Geometry: final body of the model. Coordinates: model frame, mm. Coordinates: 2 decimals unless noted, no trailing zeros. Order: outer loops, then holes, each group sorted by start corner. A loop starts at its lowest first (then second) coordinate and runs counter-clockwise, first axis right, second up. Notation, with made-up numbers: (46.5, 3.25) -> (102.5, 3.25) arc R22 cw to (102.5, 11.25) -> close; hole circle Ø6 at (20.25, -8). An arc over 180 degrees is marked (long way). Use one line per item in the form item = value.
Autodesk Fusion 360 part; units mm, degrees
sketch "Dog_body" plane through (0, 0, 0) normal (0, 0, 1) x (1, 0, 0)
  line L0 (-5.9546, 3.7769) -> (-5.6, 3.7769)
  line L1 (-5.6, 3.7769) -> (-5.6, 4.1551)
  line L2 (-5.6, 4.1551) -> (-5.2, 4.1551)
  line L3 (-5.2, 4.1551) -> (-5.2, 4.6)
  line L4 (-5.2, 4.6) -> (-4.8, 4.6)
  line L5 (-4.8, 4.6) -> (-4.8, 5)
  line L6 (-4.8, 5) -> (-4.0585, 5)
  line L7 (-4.0585, 5) -> (-4.0585, 5.4)
  line L8 (-4.0585, 5.4) -> (-2.4, 5.4)
  line L9 (-2.4, 5.4) -> (-2.4, 5)
  line L10 (-2.4, 5) -> (-0.4, 5)
  line L11 (-0.4, 5) -> (-0.4, 4.6)
  line L12 (-5.9546, 3.7769) -> (-5.9546, 2.2)
  line L13 (-5.9546, 2.2) -> (-5.6, 2.2)
  line L14 (-5.6, 2.2) -> (-5.6, 1.4)
  line L15 (-5.6, 1.4) -> (-5.9546, 1.4)
  line L16 (-5.9546, 1.4) -> (-5.9546, 0.2)
  line L17 (-5.9546, 0.2) -> (-5.6, 0.2)
  line L18 (-5.6, 0.2) -> (-5.6, -0.2)
  line L19 (-5.6, -0.2) -> (-4.8, -0.2)
  line L20 (-4.8, -0.2) -> (-4.8, -0.7)
  line L21 (-4.8, -0.7) -> (-3.6, -0.7)
  line L22 (-3.6, -0.7) -> (-3.6, -1.9)
  line L23 (-3.6, -1.9) -> (-3.2, -1.9)
  line L24 (-3.2, -1.9) -> (-3.2, -3)
  line L25 (-3.2, -3) -> (-3.6, -3)
  line L26 (-3.6, -3) -> (-3.6, -3.7529)
  line L27 (-3.6, -3.7529) -> (-4.1, -3.7529)
  line L28 (-4.1, -3.7529) -> (-4.1, -4.6)
  line L29 (-4.1, -4.6) -> (-2.4, -4.6)
  line L30 (-2.4, -4.6) -> (-2.4, -4.1765)
  line L31 (-2.4, -4.1765) -> (-1.9, -4.1765)
  line L32 (-1.9, -4.1765) -> (-1.9, -3.4)
  line L33 (-1.9, -3.4) -> (-1.1, -3.4)
  line L34 (-1.1, -3.4) -> (-1.1, -4.1765)
  line L35 (-1.1, -4.1765) -> (-1.6, -4.1765)
  line L36 (-1.6, -4.1765) -> (-1.6, -5)
  line L37 (-1.6, -5) -> (-0.1, -5)
  line L38 (-0.1, -5) -> (-0.1, -4.5882)
  line L39 (-0.1, -4.5882) -> (0.5, -4.5882)
  line L40 (0.5, -4.5882) -> (0.5, -3.8)
  line L41 (5.1495, 3.3539) -> (5.1495, 1.4)
  line L42 (5.1495, 1.4) -> (4.8, 1.4)
  line L43 (4.8, 1.4) -> (4.8, 1)
  line L44 (4.8, 1) -> (5.1495, 1)
  line L45 (5.1495, 1) -> (5.1495, 0.2)
  line L46 (5.1495, 0.2) -> (5.5479, 0.2)
  line L47 (5.5479, 0.2) -> (5.5479, -1)
  line L48 (5.5479, -1) -> (5.9, -1)
  line L49 (5.9, -1) -> (5.9, -3.4)
  line L50 (-0.4, 4.6) -> (0, 4.6)
  line L51 (0, 4.6) -> (0, 4.2)
  line L52 (0, 4.2) -> (0.4, 4.2)
  line L53 (0.4, 4.2) -> (0.4, 3.8)
  line L54 (0.4, 3.8) -> (0.8, 3.8)
  line L55 (0.8, 3.8) -> (0.8, 3.4)
  line L56 (0.8, 3.4) -> (1.2, 3.4)
  line L57 (1.2, 3.4) -> (1.2, 1.8)
  line L58 (1.2, 1.8) -> (0.8, 1.8)
  line L59 (0.8, 1.8) -> (0.8, 1.4)
  line L60 (0.8, 1.4) -> (0.4, 1.4)
  line L61 (0.4, 1.4) -> (0.4, 1)
  line L62 (0.4, 1) -> (1.1786, 1)
  line L63 (1.1786, 1) -> (1.1786, 1.4)
  line L64 (1.1786, 1.4) -> (1.9689, 1.4)
  line L65 (1.9689, 1.4) -> (1.9689, 1.8)
  line L66 (1.9689, 1.8) -> (3.6, 1.8)
  line L67 (3.6, 1.8) -> (3.6, 2.2)
  line L68 (3.6, 2.2) -> (4, 2.2)
  line L69 (4, 2.2) -> (4, 3.3596)
  line L70 (4, 3.3596) -> (3.5503, 3.3596)
  line L71 (3.5503, 3.3596) -> (3.5503, 4.2)
  line L72 (3.5503, 4.2) -> (3.2, 4.2)
  line L73 (3.2, 4.2) -> (3.2, 5)
  line L74 (3.2, 5) -> (4, 5)
  line L75 (4, 5) -> (4, 4.6)
  line L76 (4, 4.6) -> (4.4, 4.6)
  line L77 (4.4, 4.6) -> (4.4, 4.2)
  line L78 (4.4, 4.2) -> (4.7373, 4.2)
  line L79 (4.7373, 4.2) -> (4.7373, 3.4)
  line L80 (4.7373, 3.4) -> (4.7373, 3.3539)
  line L81 (4.7373, 3.3539) -> (5.1495, 3.3539)
  line L82 (0.5, -3.8) -> (0.8, -3.8)
  line L83 (0.8, -3.8) -> (0.8, -3)
  line L84 (0.8, -3) -> (1.5654, -3)
  line L85 (1.5654, -3) -> (1.5654, -3.5)
  line L86 (1.5654, -3.5) -> (3.2, -3.5)
  line L87 (3.2, -3.5) -> (3.2, -2.6)
  line L88 (3.2, -2.6) -> (3.6, -2.6)
  line L89 (3.6, -2.6) -> (3.6, -2.2)
  line L90 (3.6, -2.2) -> (4.3564, -2.2)
  line L91 (4.3564, -2.2) -> (4.3564, -2.9)
  line L92 (4.3564, -2.9) -> (3.9, -2.9)
  line L93 (3.9, -2.9) -> (3.9, -3.8)
  line L94 (3.9, -3.8) -> (5.5, -3.8)
  line L95 (5.5, -3.4) -> (5.9, -3.4)
  line L96 (5.5, -3.4) -> (5.5, -3.8)
extrude "Extrude1" add sketch "Dog_body" along normal blind 0.5
sketch "Dog_eyes" plane through (0, 0, 0.5) normal (0, 0, 1) x (-1, 0, 0)
  line L0 (5.9546, -3.7769) -> (5.9546, -2.2)
  line L1 (5.9546, -2.2) -> (5.6, -2.2)
  line L2 (5.6, -2.2) -> (5.6, -1.4)
  line L3 (5.6, -1.4) -> (5.9546, -1.4)
  line L4 (5.9546, -1.4) -> (5.9546, -0.2)
  line L5 (5.9546, -0.2) -> (5.6, -0.2)
  line L6 (5.6, -0.2) -> (5.6, 0.2)
  line L7 (5.6, 0.2) -> (4.8, 0.2)
  line L8 (4.8, 0.2) -> (4.8, 0.7)
  line L9 (4.8, 0.7) -> (3.6, 0.7)
  line L10 (3.6, 0.7) -> (3.6, 1.9)
  line L11 (3.6, 1.9) -> (3.2, 1.9)
  line L12 (3.2, 1.9) -> (3.2, 3)
  line L13 (3.2, 3) -> (3.6, 3)
  line L14 (3.6, 3) -> (3.6, 3.7529)
  line L15 (3.6, 3.7529) -> (4.1, 3.7529)
  line L16 (4.1, 3.7529) -> (4.1, 4.6)
  line L17 (4.1, 4.6) -> (2.4, 4.6)
  line L18 (2.4, 4.6) -> (2.4, 4.1765)
  line L19 (2.4, 4.1765) -> (1.9, 4.1765)
  line L20 (1.9, 4.1765) -> (1.9, 3.4)
  line L21 (1.9, 3.4) -> (1.1, 3.4)
  line L22 (1.1, 3.4) -> (1.1, 4.1765)
  line L23 (1.1, 4.1765) -> (1.6, 4.1765)
  line L24 (1.6, 4.1765) -> (1.6, 5)
  line L25 (1.6, 5) -> (0.1, 5)
  line L26 (0.1, 5) -> (0.1, 4.5882)
  line L27 (0.1, 4.5882) -> (-0.5, 4.5882)
  line L28 (-0.5, 4.5882) -> (-0.5, 3.8)
  line L29 (-0.5, 3.8) -> (-0.8, 3.8)
  line L30 (-0.8, 3.8) -> (-0.8, 3)
  line L31 (-0.8, 3) -> (-1.5654, 3)
  line L32 (-1.5654, 3) -> (-1.5654, 3.5)
  line L33 (-1.5654, 3.5) -> (-3.2, 3.5)
  line L34 (-3.2, 3.5) -> (-3.2, 2.6)
  line L35 (-3.2, 2.6) -> (-3.6, 2.6)
  line L36 (-3.6, 2.6) -> (-3.6, 2.2)
  line L37 (-3.6, 2.2) -> (-4.3564, 2.2)
  line L38 (-4.3564, 2.2) -> (-4.3564, 2.9)
  line L39 (-4.3564, 2.9) -> (-3.9, 2.9)
  line L40 (-3.9, 2.9) -> (-3.9, 3.8)
  line L41 (-3.9, 3.8) -> (-5.5, 3.8)
  line L42 (-5.5, 3.8) -> (-5.5, 3.4)
  line L43 (-5.5, 3.4) -> (-5.9, 3.4)
  line L44 (-5.9, 3.4) -> (-5.9, 1)
  line L45 (-5.9, 1) -> (-5.5479, 1)
  line L46 (-5.5479, 1) -> (-5.5479, -0.2)
  line L47 (-5.5479, -0.2) -> (-5.1495, -0.2)
  line L48 (-5.1495, -0.2) -> (-5.1495, -1)
  line L49 (-5.1495, -1) -> (-4.8, -1)
  line L50 (-4.8, -1) -> (-4.8, -1.4)
  line L51 (-4.8, -1.4) -> (-5.1495, -1.4)
  line L52 (-5.1495, -1.4) -> (-5.1495, -3.3539)
  line L53 (-5.1495, -3.3539) -> (-4.7373, -3.3539)
  line L54 (-4.7373, -3.3539) -> (-4.7373, -4.2)
  line L55 (-4.7373, -4.2) -> (-4.4, -4.2)
  line L56 (-4.4, -4.2) -> (-4.4, -4.6)
  line L57 (-4.4, -4.6) -> (-4, -4.6)
  line L58 (-4, -4.6) -> (-4, -5)
  line L59 (-4, -5) -> (-3.2, -5)
  line L60 (-3.2, -5) -> (-3.2, -4.2)
  line L61 (-3.2, -4.2) -> (-3.5503, -4.2)
  line L62 (-3.5503, -4.2) -> (-3.5503, -3.3596)
  line L63 (-3.5503, -3.3596) -> (-4, -3.3596)
  line L64 (-4, -3.3596) -> (-4, -2.2)
  line L65 (-4, -2.2) -> (-3.6, -2.2)
  line L66 (-3.6, -2.2) -> (-3.6, -1.8)
  line L67 (-3.6, -1.8) -> (-1.9689, -1.8)
  line L68 (-1.9689, -1.8) -> (-1.9689, -1.4)
  line L69 (-1.9689, -1.4) -> (-1.1786, -1.4)
  line L70 (-1.1786, -1.4) -> (-1.1786, -1)
  line L71 (-1.1786, -1) -> (-0.4, -1)
  line L72 (-0.4, -1) -> (-0.4, -1.4)
  line L73 (-0.4, -1.4) -> (-0.8, -1.4)
  line L74 (-0.8, -1.4) -> (-0.8, -1.8)
  line L75 (-0.8, -1.8) -> (-1.2, -1.8)
  line L76 (-1.2, -1.8) -> (-1.2, -3.4)
  line L77 (-1.2, -3.4) -> (-0.8, -3.4)
  line L78 (-0.8, -3.4) -> (-0.8, -3.8)
  line L79 (-0.8, -3.8) -> (-0.4, -3.8)
  line L80 (-0.4, -3.8) -> (-0.4, -4.2)
  line L81 (-0.4, -4.2) -> (0, -4.2)
  line L82 (0, -4.2) -> (0, -4.6)
  line L83 (0, -4.6) -> (0.4, -4.6)
  line L84 (0.4, -4.6) -> (0.4, -5)
  line L85 (0.4, -5) -> (2.4, -5)
  line L86 (2.4, -5) -> (2.4, -5.4)
  line L87 (2.4, -5.4) -> (4.0585, -5.4)
  line L88 (4.0585, -5.4) -> (4.0585, -5)
  line L89 (4.0585, -5) -> (4.8, -5)
  line L90 (4.8, -5) -> (4.8, -4.6)
  line L91 (4.8, -4.6) -> (5.2, -4.6)
  line L92 (5.2, -4.6) -> (5.2, -4.1551)
  line L93 (5.2, -4.1551) -> (5.6, -4.1551)
  line L94 (5.6, -4.1551) -> (5.6, -3.7769)
  line L95 (5.6, -3.7769) -> (5.9546, -3.7769)
  line L96 (3.2, -3) -> (3.2, -2)
  line L97 (3.2, -2) -> (2.6, -2)
  line L98 (2.6, -2) -> (2.6, -3)
  line L99 (2.6, -3) -> (3.2, -3)
  line L100 (5.2, -3.3) -> (5.2, -2.5)
  line L101 (5.2, -2.5) -> (4.8, -2.5)
  line L102 (4.8, -2.5) -> (4.8, -3.4)
  line L103 (4.8, -3.4) -> (5.2, -3.4)
  line L104 (5.2, -3.4) -> (5.2, -3.3)
extrude "Extrude2" cut sketch "Dog_eyes" against normal blind 0.2 contours L96 L97 L98 L99 | L100 L101 L102 L103 L104
sketch "Sketch3" plane through (0, 0, 0.5) normal (0, 0, 1) x (-1, 0, 0)
  line L0 (4.8, -2.5) -> (5.2, -2.5)
  line L1 (5.2, -2.5) -> (5.2, -3.4)
  line L2 (5.2, -3.4) -> (4.8, -3.4)
  line L3 (4.8, -3.4) -> (4.8, -2.5)
  line L4 (3.2, -2) -> (3.2, -3)
  line L5 (3.2, -3) -> (2.6, -3)
  line L6 (2.6, -3) -> (2.6, -2)
  line L7 (2.6, -2) -> (3.2, -2)
  line L8 (5.9546, -3.7769) -> (5.9546, -2.2)
  line L9 (5.9546, -2.2) -> (5.6, -2.2)
  line L10 (5.6, -2.2) -> (5.6, -1.4)
  line L11 (5.6, -1.4) -> (5.9546, -1.4)
  line L12 (5.9546, -1.4) -> (5.9546, -0.2)
  line L13 (5.9546, -0.2) -> (5.6, -0.2)
  line L14 (5.6, -0.2) -> (5.6, 0.2)
  line L15 (5.6, 0.2) -> (4.8, 0.2)
  line L16 (4.8, 0.2) -> (4.8, 0.7)
  line L17 (4.8, 0.7) -> (3.6, 0.7)
  line L18 (3.6, 0.7) -> (3.6, 1.9)
  line L19 (3.6, 1.9) -> (3.2, 1.9)
  line L20 (3.2, 1.9) -> (3.2, 3)
  line L21 (3.2, 3) -> (3.6, 3)
  line L22 (3.6, 3) -> (3.6, 3.7529)
  line L23 (3.6, 3.7529) -> (4.1, 3.7529)
  line L24 (4.1, 3.7529) -> (4.1, 4.6)
  line L25 (4.1, 4.6) -> (2.4, 4.6)
  line L26 (2.4, 4.6) -> (2.4, 4.1765)
  line L27 (2.4, 4.1765) -> (1.9, 4.1765)
  line L28 (1.9, 4.1765) -> (1.9, 3.4)
  line L29 (1.9, 3.4) -> (1.1, 3.4)
  line L30 (1.1, 3.4) -> (1.1, 4.1765)
  line L31 (1.1, 4.1765) -> (1.6, 4.1765)
  line L32 (1.6, 4.1765) -> (1.6, 5)
  line L33 (1.6, 5) -> (0.1, 5)
  line L34 (0.1, 5) -> (0.1, 4.5882)
  line L35 (0.1, 4.5882) -> (-0.5, 4.5882)
  line L36 (-0.5, 4.5882) -> (-0.5, 3.8)
  line L37 (-0.5, 3.8) -> (-0.8, 3.8)
  line L38 (-0.8, 3.8) -> (-0.8, 3)
  line L39 (-0.8, 3) -> (-1.5654, 3)
  line L40 (-1.5654, 3) -> (-1.5654, 3.5)
  line L41 (-1.5654, 3.5) -> (-3.2, 3.5)
  line L42 (-3.2, 3.5) -> (-3.2, 2.6)
  line L43 (-3.2, 2.6) -> (-3.6, 2.6)
  line L44 (-3.6, 2.6) -> (-3.6, 2.2)
  line L45 (-3.6, 2.2) -> (-4.3564, 2.2)
  line L46 (-4.3564, 2.2) -> (-4.3564, 2.9)
  line L47 (-4.3564, 2.9) -> (-3.9, 2.9)
  line L48 (-3.9, 2.9) -> (-3.9, 3.8)
  line L49 (-3.9, 3.8) -> (-5.5, 3.8)
  line L50 (-5.5, 3.8) -> (-5.5, 3.4)
  line L51 (-5.5, 3.4) -> (-5.9, 3.4)
  line L52 (-5.9, 3.4) -> (-5.9, 1)
  line L53 (-5.9, 1) -> (-5.5479, 1)
  line L54 (-5.5479, 1) -> (-5.5479, -0.2)
  line L55 (-5.5479, -0.2) -> (-5.1495, -0.2)
  line L56 (-5.1495, -0.2) -> (-5.1495, -1)
  line L57 (-5.1495, -1) -> (-4.8, -1)
  line L58 (-4.8, -1) -> (-4.8, -1.4)
  line L59 (-4.8, -1.4) -> (-5.1495, -1.4)
  line L60 (-5.1495, -1.4) -> (-5.1495, -3.3539)
  line L61 (-5.1495, -3.3539) -> (-4.7373, -3.3539)
  line L62 (-4.7373, -3.3539) -> (-4.7373, -4.2)
  line L63 (-4.7373, -4.2) -> (-4.4, -4.2)
  line L64 (-4.4, -4.2) -> (-4.4, -4.6)
  line L65 (-4.4, -4.6) -> (-4, -4.6)
  line L66 (-4, -4.6) -> (-4, -5)
  line L67 (-4, -5) -> (-3.2, -5)
  line L68 (-3.2, -5) -> (-3.2, -4.2)
  line L69 (-3.2, -4.2) -> (-3.5503, -4.2)
  line L70 (-3.5503, -4.2) -> (-3.5503, -3.3596)
  line L71 (-3.5503, -3.3596) -> (-4, -3.3596)
  line L72 (-4, -3.3596) -> (-4, -2.2)
  line L73 (-4, -2.2) -> (-3.6, -2.2)
  line L74 (-3.6, -2.2) -> (-3.6, -1.8)
  line L75 (-3.6, -1.8) -> (-1.9689, -1.8)
  line L76 (-1.9689, -1.8) -> (-1.9689, -1.4)
  line L77 (-1.9689, -1.4) -> (-1.1786, -1.4)
  line L78 (-1.1786, -1.4) -> (-1.1786, -1)
  line L79 (-1.1786, -1) -> (-0.4, -1)
  line L80 (-0.4, -1) -> (-0.4, -1.4)
  line L81 (-0.4, -1.4) -> (-0.8, -1.4)
  line L82 (-0.8, -1.4) -> (-0.8, -1.8)
  line L83 (-0.8, -1.8) -> (-1.2, -1.8)
  line L84 (-1.2, -1.8) -> (-1.2, -3.4)
  line L85 (-1.2, -3.4) -> (-0.8, -3.4)
  line L86 (-0.8, -3.4) -> (-0.8, -3.8)
  line L87 (-0.8, -3.8) -> (-0.4, -3.8)
  line L88 (-0.4, -3.8) -> (-0.4, -4.2)
  line L89 (-0.4, -4.2) -> (0, -4.2)
  line L90 (0, -4.2) -> (0, -4.6)
  line L91 (0, -4.6) -> (0.4, -4.6)
  line L92 (0.4, -4.6) -> (0.4, -5)
  line L93 (0.4, -5) -> (2.4, -5)
  line L94 (2.4, -5) -> (2.4, -5.4)
  line L95 (2.4, -5.4) -> (4.0585, -5.4)
  line L96 (4.0585, -5.4) -> (4.0585, -5)
  line L97 (4.0585, -5) -> (4.8, -5)
  line L98 (4.8, -5) -> (4.8, -4.6)
  line L99 (4.8, -4.6) -> (5.2, -4.6)
  line L100 (5.2, -4.6) -> (5.2, -4.1551)
  line L101 (5.2, -4.1551) -> (5.6, -4.1551)
  line L102 (5.6, -4.1551) -> (5.6, -3.7769)
  line L103 (5.6, -3.7769) -> (5.9546, -3.7769)
  line L104 (5.6, -1.4) -> (4.4, -1.4)
  line L105 (4.4, -1.4) -> (4.4, -0.6)
  line L106 (4.4, -0.6) -> (5.9546, -0.6)
  line L107 (5.9546, -1.4) -> (5.5, -1.4)
  line L108 (5.6, -1.4) -> (5.9546, -1.4)
  line L109 (5.6, -1.4) -> (4.4, -1.4)
  line L110 (5.6, -1.4) -> (5.9546, -1.4)
  line L111 (5.9546, -0.6568) -> (5.9546, -0.6)
  line L112 (5.9546, -0.6) -> (5.9546, -1.4)
extrude "Extrude3" add sketch "Sketch3" along normal blind 0.2 contours L11 L12 L104 L105 L106 L107 L108 L109 L110 L111 L112
extrude "Extrude4" cut 1 faces at (-4.9182, 0.8667, 0.7) along direction (0, 0, -1) blind 0.1
hole "Hole1" at (-3.4028, 4.5934, 0.5) direction (0, 0, -1) diameter 1 depth 2.5 tip angle 118
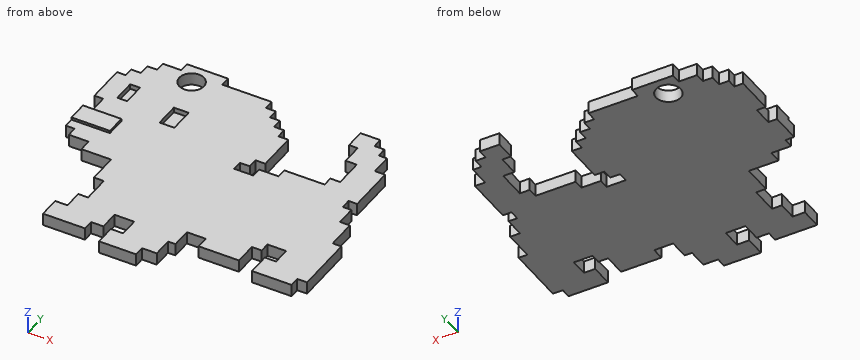
1) Section A-A, the plane y = 2.75. Output: boundary loops of the cut face in (x, z).
Results found:
outline = (-5.95, 0) -> (1.2, 0) -> (1.2, 0.5) -> (-2.6, 0.5) -> (-2.6, 0.3) -> (-3.2, 0.3) -> (-3.2, 0.5) -> (-4.8, 0.5) -> (-4.8, 0.3) -> (-5.2, 0.3) -> (-5.2, 0.5) -> (-5.95, 0.5) -> close; (4, 0) -> (5.15, 0) -> (5.15, 0.5) -> (4, 0.5) -> close
2) Section D-D, the plane z = 0.4. Give the number of separate pieces and of enclosed holes in the cut face, and give its area (3 significant figures).
Results found:
separate_pieces = 1
enclosed_holes = 3
area = 78.9 mm2
3) Material intervals for probe 1 along Y at (x, z) = (3.5, 0.25); probe 2 along X at (y, z) = (4.75, 0.45); probe 3 along Y at (x, z) = (1, 0.1), sorted ascending. Write a range as from..to.
Results found:
probe_1 = -2.6..1.8, 4.2..5
probe_2 = -4.8..-3.88, -2.93..-0.4, 3.2..4
probe_3 = -3..1, 1.8..3.4
4) Section C-C, the plane x = 2.75. Output: boundary loops of the cut face in (y, z), and give its area (3 significant figures).
Results found:
outline = (-3.5, 0) -> (1.8, 0) -> (1.8, 0.5) -> (-3.5, 0.5) -> close
area = 2.65 mm2
5) Section B-B, the plane y = 0. Output: boundary loops of the cut face in (x, z), and give its area (3 significant figures).
Results found:
outline = (-5.6, 0) -> (5.55, 0) -> (5.55, 0.5) -> (-5.6, 0.5) -> close
area = 5.57 mm2
6) Contact query for flat-ended pins moving along their axis: P1, Ø0.5, axis at x = -3, y = 2.5, coming from the +Z side; P2, Ø1, axis at x = -2.5, y = -0.5, coming from the -Z side. Output: stop coordinate, or through.
Results found:
P1 = 0.5
P2 = 0
